Source: CAD feature listing. Evaluate the final solid. Frame: model axes, mm. Face numbers are marked on the shaded views. A direction names the side the tool comes from. Round coordinates to 2 decimals unless told otherwise and drop trailing zeros. Order: outer loops, then holes, each group sorted by start corner. A loop starts at its lowest first (then second) coordinate and runs counter-clockwise, first axis right, second up. Notation, with made-up numbers: (-19.5, 49) - (26.5, 49) arc R18 cw to (26.5, 65) - close; hole circle Ø5 at (64, 0.5). An arc over 180 degrees is marked (long way). Return JSON: item names as keys, results as strings. Group by question number.
1) Access query for the marked faces 1 and 2. Directions: +Z, -Z, +X, -X, +Y, -Y. A direction counts if a zero-diameter tool reaches every point of the face in a straight line with its end or side. Return the directions, or none.
2) Mould query, pull axis Z, two halves, no side actions, for the marked faces 3, 4, 5 and 6. Classes: pulls with the +Z half, pulls with the -Z half, needs draft (parallel to the pull), parting line crosses it, or undercut.
3) Section C-C, the plane y = 22. Give the number of separate pieces and of enclosed holes in the cut face, plus the area to 3 significant figures.
4) Ray query, line 1 (X direction, y = 12.5, z = -75.25); line 2 (X direction, y = 23.75, z = -38); line 3 (Z direction, x = 14.5, y = 12.5). Return the intervals inside material, ascending. Write a range as from..to.
5) Section A-A, the plane x = 62. Return loops of the section in (y, z).
6) Section D-D, the plane x = 30.5. Return loops of the section in (y, z).
7) Section B-B, the plane z = -24. Return loops of the section in (x, y), plus the area to 3 significant figures.
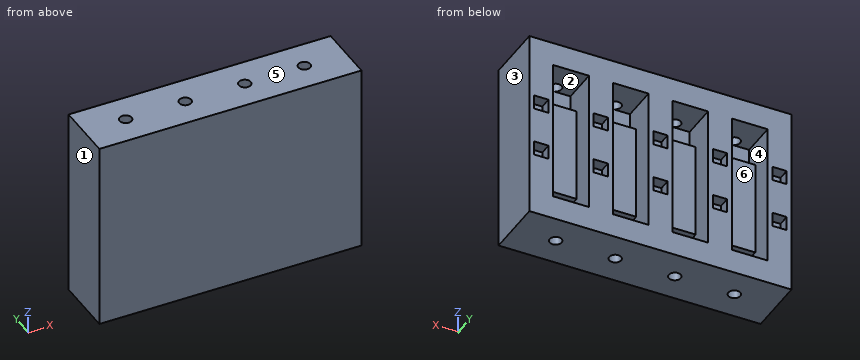
```python
from build123d import *

# Parameters (mm, degrees)
SKETCH1_W           = 110
SKETCH1_H           = 25
BOSS_EXTRUDE1_DEPTH = 80
SKETCH2_W           = 15
SKETCH2_H           = 10
CUT_EXTRUDE1_DEPTH  = 15
SKETCH4_R           = 2.5
CUT_EXTRUDE2_DEPTH  = 10
SKETCH5_W           = 15
SKETCH5_H           = 40
CUT_EXTRUDE3_DEPTH  = 10
SKETCH6_W           = 6
SKETCH6_H           = 6
CUT_EXTRUDE4_DEPTH  = 5


with BuildPart() as part:
    # Sketch1 → Boss-Extrude1 (new body)
    with BuildSketch(Plane.XY):
        with Locations((55, 12.5)):
            Rectangle(SKETCH1_W, SKETCH1_H)
    extrude(amount=-BOSS_EXTRUDE1_DEPTH)

    # Sketch2 → Cut-Extrude1 (cut)
    with BuildSketch(Plane(origin=(0, 25, 0), x_dir=(1, 0, 0), z_dir=(0, 1, 0))):
        with Locations((17.5, 15)):
            Rectangle(SKETCH2_W, SKETCH2_H)
        with Locations((17.5, 65)):
            Rectangle(SKETCH2_W, SKETCH2_H)
        with Locations((42.5, 15)):
            Rectangle(SKETCH2_W, SKETCH2_H)
        with Locations((42.5, 65)):
            Rectangle(SKETCH2_W, SKETCH2_H)
        with Locations((67.5, 15)):
            Rectangle(SKETCH2_W, SKETCH2_H)
        with Locations((67.5, 65)):
            Rectangle(SKETCH2_W, SKETCH2_H)
        with Locations((92.5, 15)):
            Rectangle(SKETCH2_W, SKETCH2_H)
        with Locations((92.5, 65)):
            Rectangle(SKETCH2_W, SKETCH2_H)
    extrude(amount=-CUT_EXTRUDE1_DEPTH, mode=Mode.SUBTRACT)

    # Sketch4 → Cut-Extrude2 (cut)
    with BuildSketch(Plane.XY):
        with Locations((17.5, 12.5)):
            Circle(SKETCH4_R)
        with Locations((42.5, 12.5)):
            Circle(SKETCH4_R)
        with Locations((67.5, 12.5)):
            Circle(SKETCH4_R)
        with Locations((92.5, 12.5)):
            Circle(SKETCH4_R)
    cut_extrude2 = extrude(amount=-CUT_EXTRUDE2_DEPTH, mode=Mode.SUBTRACT)

    # Mirror1: Cut-Extrude2 across plane
    add(cut_extrude2.mirror(Plane.XY.offset(-40)), mode=Mode.SUBTRACT)

    # Sketch5 → Cut-Extrude3 (cut)
    with BuildSketch(Plane(origin=(0, 25, 0), x_dir=(1, 0, 0), z_dir=(0, 1, 0))):
        with Locations((42.5, 40)):
            Rectangle(SKETCH5_W, SKETCH5_H)
        with Locations((17.5, 40)):
            Rectangle(SKETCH5_W, SKETCH5_H)
        with Locations((67.5, 40)):
            Rectangle(SKETCH5_W, SKETCH5_H)
        with Locations((92.5, 40)):
            Rectangle(SKETCH5_W, SKETCH5_H)
    extrude(amount=-CUT_EXTRUDE3_DEPTH, mode=Mode.SUBTRACT)

    # Sketch6 → Cut-Extrude4 (cut)
    with BuildSketch(Plane(origin=(0, 25, 0), x_dir=(1, 0, 0), z_dir=(0, 1, 0))):
        with Locations((5, 50.5)):
            Rectangle(SKETCH6_W, SKETCH6_H)
        with Locations((30, 50.5)):
            Rectangle(SKETCH6_W, SKETCH6_H)
        with Locations((55, 50.5)):
            Rectangle(SKETCH6_W, SKETCH6_H)
        with Locations((80, 50.5)):
            Rectangle(SKETCH6_W, SKETCH6_H)
        with Locations((105, 50.5)):
            Rectangle(SKETCH6_W, SKETCH6_H)
        with Locations((30, 29.5)):
            Rectangle(SKETCH6_W, SKETCH6_H)
        with Locations((55, 29.5)):
            Rectangle(SKETCH6_W, SKETCH6_H)
        with Locations((80, 29.5)):
            Rectangle(SKETCH6_W, SKETCH6_H)
        with Locations((105, 29.5)):
            Rectangle(SKETCH6_W, SKETCH6_H)
        with Locations((5, 29.5)):
            Rectangle(SKETCH6_W, SKETCH6_H)
    extrude(amount=-CUT_EXTRUDE4_DEPTH, mode=Mode.SUBTRACT)


solid = part.part
```
Geometry check:
{
 "1": {"face 1": "+Z, -Z, -X, +Y, -Y", "face 2": "+Y"},
 "2": {"face 3": "needs draft", "face 4": "undercut", "face 5": "pulls with the +Z half", "face 6": "undercut"},
 "3": {"separate pieces": "1", "enclosed holes": "14", "area": "4,840 mm2"},
 "4": {"line 1": "0..15, 20..40, 45..65, 70..90, 95..110", "line 2": "0..10, 25..35, 50..60, 75..85, 100..110", "line 3": "-80..-70, -60..-20, -10..0"},
 "5": {"outline": "(0, -80) - (25, -80) - (25, -70) - (10, -70) - (10, -60) - (15, -60) - (15, -20) - (10, -20) - (10, -10) - (25, -10) - (25, 0) - (0, 0) - close"},
 "6": {"outline": "(0, -80) - (25, -80) - (25, -53.5) - (20, -53.5) - (20, -47.5) - (25, -47.5) - (25, -32.5) - (20, -32.5) - (20, -26.5) - (25, -26.5) - (25, 0) - (0, 0) - close"},
 "7": {"outline": "(0, 0) - (110, 0) - (110, 25) - (100, 25) - (100, 15) - (85, 15) - (85, 25) - (75, 25) - (75, 15) - (60, 15) - (60, 25) - (50, 25) - (50, 15) - (35, 15) - (35, 25) - (25, 25) - (25, 15) - (10, 15) - (10, 25) - (0, 25) - close", "area": "2,150 mm2"}
}
